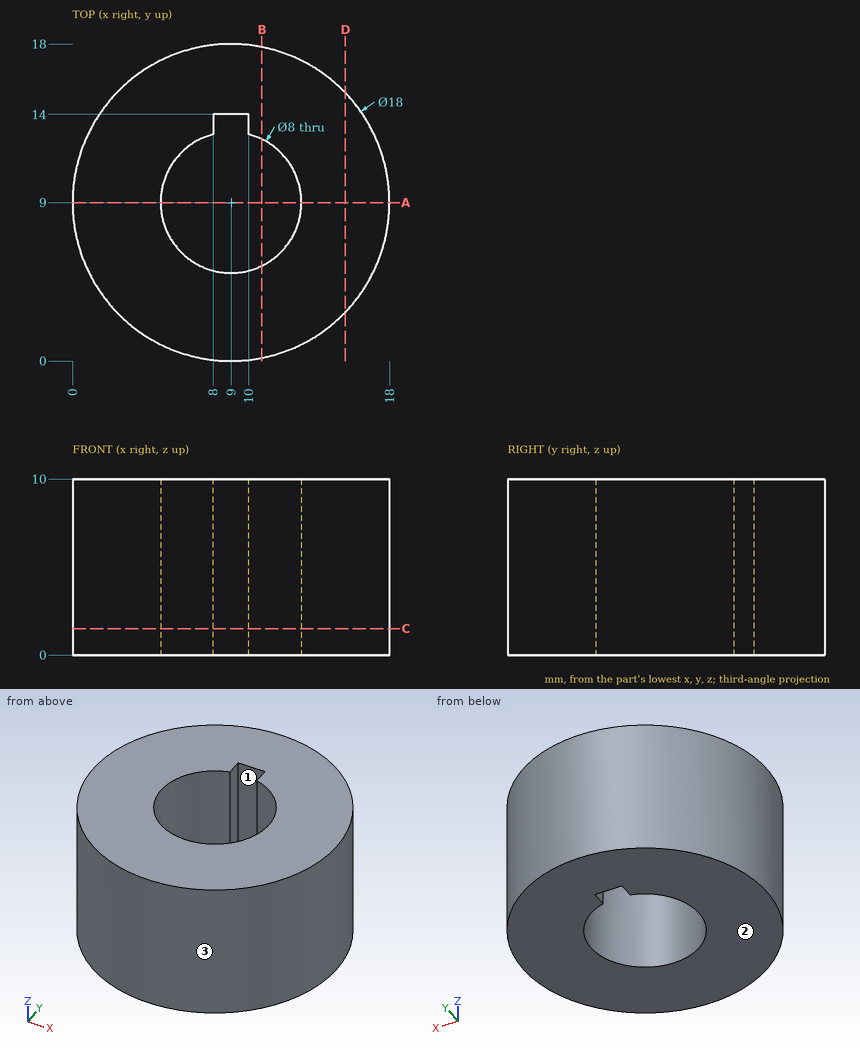
The figure shows three views and two pictorial views of one solid part (mm, origin at its lowest corner). Answer the questions. Round coordinates to 2 decimals unless told otherwise and drop trailing zeros. Order: outer loops, then holes, each group sorted by start corner. A loop starts at its lowest first (then second) coordinate and runs counter-clockwise, first axis right, second up. Notation, with made-up numbers: M 49.25,15.5 L 53.25,15.5 A11 ccw 53.25,33.5 Z; hole C 49.5,80 d9. An arc over 180 degrees is marked long. Put each result on its own line as item: value. Start each with the question number.
Q1. Straight lines are drawn through the part: L1, parallel to Y at x = 9, z = 4; L2, parallel to Y at x = 10.75, z = 9.5; L3, parallel to X at y = 10.5, z = 2.75. For each, find the intervals that lie inside material, in ascending order. Write a range as [from, to].
Q2. Section C-C, the plane z = 1.5 is taken. Write down the section's boundary in (x, y).
Q3. Section A-A, the plane y = 9 is taken. Write down the section's boundary in (x, z).
Q4. Section D-D, the plane x = 15.5 is taken. Write down the section's boundary in (y, z), and give its area (3 significant figures).
Q5. Section B-B, the plane x = 10.75 is taken. Write down the section's boundary in (y, z).
Q6. Flat-ended cylindrical pins translate along their axes: pin 1 (3 mm diameter, centred on x = 4.5, z = 3, fed in from -Y); pin 2 (2 mm diameter, centred on y = 2, z = 3.5, fed in from -X); pin 3 (0.6 mm diameter, centred on y = 13.5, z = 5, fed in from -X). Find the tip coordinate at first contact, or state that the pin passes through.
Q7. For a pull along X with two mould halves and no side action, classify the marked faces 1, 2 and 3 as pulls with the +X half, pulls with the -X half, needs draft (parallel to the pull), parting line crosses it, or undercut.
Findings below:
1. L1: y = [0, 5], [14, 18]
1. L2: y = [0.17, 5.4], [12.6, 17.83]
1. L3: x = [0.13, 5.29], [12.71, 17.87]
2. outline: C 9,9 d18; hole M 8,12.87 A4 ccw long 10,12.87 L 10,14 L 8,14 Z
3. outline: M 0,0 L 5,0 L 5,10 L 0,10 Z; M 13,0 L 18,0 L 18,10 L 13,10 Z
4. outline: M 2.78,0 L 15.22,0 L 15.22,10 L 2.78,10 Z
4. area: 124 mm^2
5. outline: M 0.17,0 L 5.4,0 L 5.4,10 L 0.17,10 Z; M 12.6,0 L 17.83,0 L 17.83,10 L 12.6,10 Z
6. pin 1: stops at y = 0.51
6. pin 2: stops at x = 2.29
6. pin 3: stops at x = 1.04
7. face 1: undercut
7. face 2: needs draft
7. face 3: parting line crosses it
